The drawing under review shows one solid part. Ordinate dimensions are in mm from its lowest x, y, z. Give positions to 0.01 mm unless a question says otherwise; leave off trailing zeros. Order: outer loops, then holes, each group sorted by start corner. A loop starts at its lowest first (then second) coordinate and runs counter-clockwise, first axis right, second up. Notation, with made-up numbers: (15, 18.5) -> (31, 18.5) arc R19 cw to (31, 46.5) -> close; hole circle Ø2 at (-23, 31.25). An arc over 180 degrees is marked (long way). One line per item, written item: value.
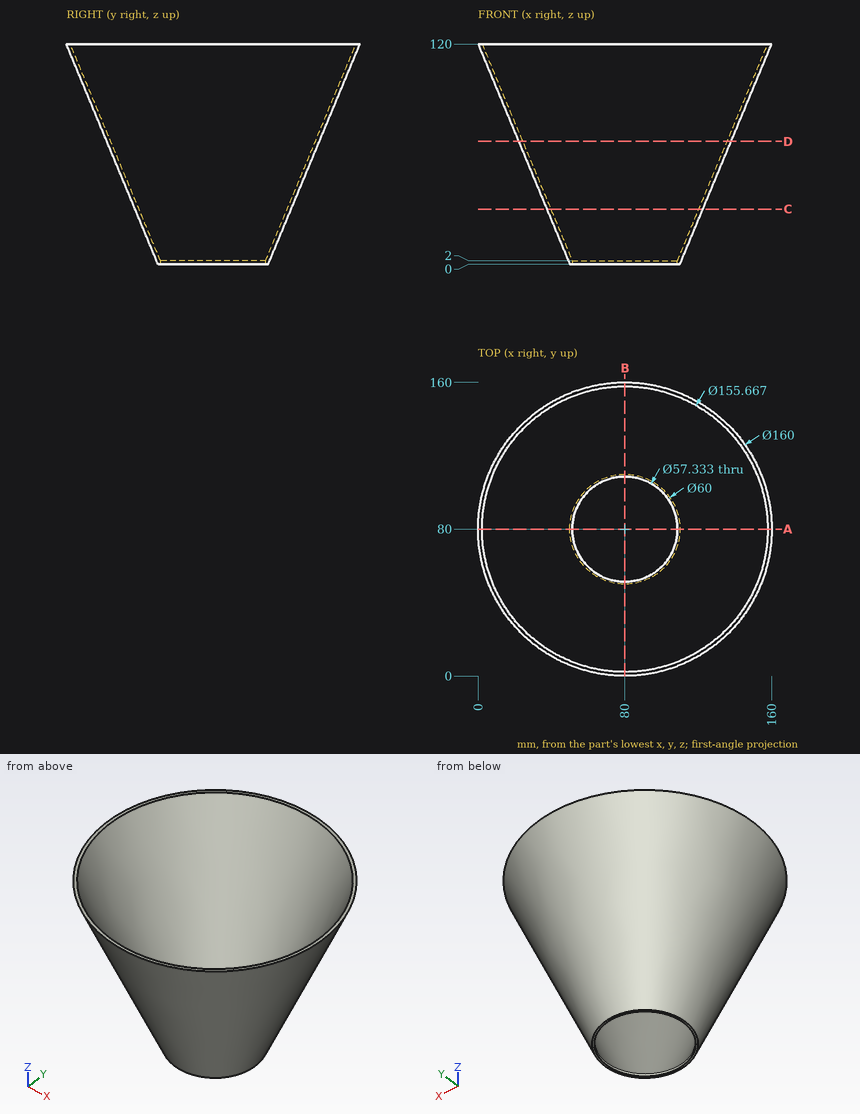
Item 1: Clearance check with flat-ended pins moving along their axes: P1, Ø3, axis at x = 42.5, z = 70, coming from the -Y side; P2, Ø2, axis at x = 133, y = 106.5, coming from the -Z side (1 decimal); P3, Ø12, axis at y = 56, z = 104.5, coming from the +X side. State where each tip first meets the part, or that it passes through.
Returned:
P1: y = 32.8
P2: z = 67.8
P3: x = 152.74
Item 2: Add section A-A on y = 80. Give the boundary of the cut face in (x, z).
Returned:
outline: (0, 120) -> (50, 0) -> (51.33, 0) -> (51.33, 2) -> (2.17, 120) -> close; (108.67, 0) -> (110, 0) -> (160, 120) -> (157.83, 120) -> (108.67, 2) -> close
Item 3: Add section D-D on z = 67. Give the boundary of the cut face in (x, y).
Returned:
outline: circle Ø115.83 at (80, 80); hole circle Ø111.5 at (80, 80)
Item 4: Add section C-C on z = 30. Give the boundary of the cut face in (x, y).
Returned:
outline: circle Ø85 at (80, 80); hole circle Ø80.67 at (80, 80)
Item 5: To check wall thickness, follow line 1 along Y through (x, z) = (97, 89); line 2 along Y through (x, z) = (80, 1); line 3 along Z through (x, y) = (139, 95) (1 decimal). State the ranges of each line that lie inside material, in increasing order. Write a range as from..to.
Returned:
line 1: 15.11..17.35, 142.65..144.89
line 2: 49.58..51.33, 108.67..110.42
line 3: 74.1..79.3
